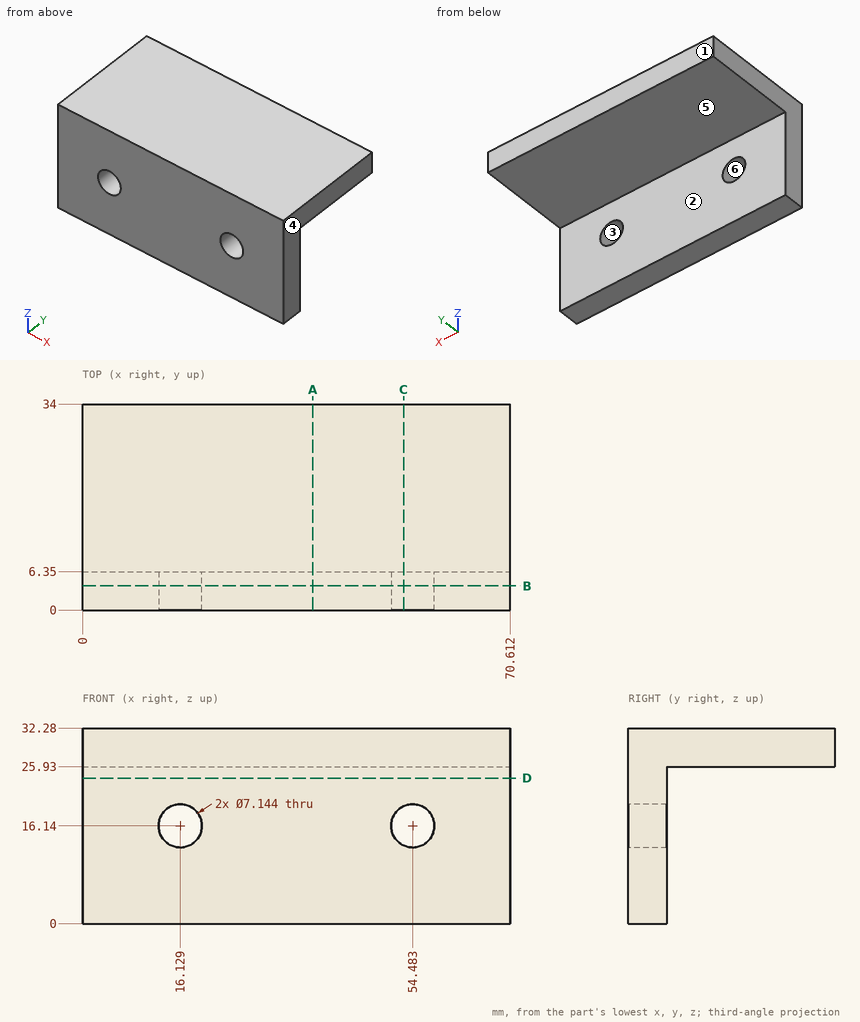
Geometry: see drawing. Coordinates: mm, zero at the bounding-box minimum. A direction names the side the tool comes from. Coordinates: 2 decimals unless noted, no trailing zeros. Loops run counter-clockwise (first coordinate to the right, second up) from the corner with the lowest first, then second, coordinate; pieces in that order, holes last. Notation, with made-up numbers: (-7, 89) - (52, 89) arc R9 cw to (52, 98) - close; hole circle Ø1 at (4, 35). An arc over 180 degrees is marked (long way). Answer in a Markdown table with one row per item.
(1) Cut plane D-D on z = 24. Output: boundary loops of the cut face in (x, y).
Model answer:
| item | result |
|---|---|
| outline | (0, 0) - (70.61, 0) - (70.61, 6.35) - (0, 6.35) - close |
(2) Mould query, pull axis X, two halves, no side actions, for the marked faces 3, 4, 5 and 6. Classes: pulls with the +X half, pulls with the -X half, needs draft (parallel to the pull), parting line crosses it, or undercut.
Model answer:
| item | result |
|---|---|
| face 3 | undercut |
| face 4 | pulls with the +X half |
| face 5 | needs draft |
| face 6 | undercut |
(3) Pin query (flat end, axial travel): P1, Ø9.5, axis at x = 54.48, z = 16.14, coming from the +Y side; P2, Ø8.5, axis at x = 28.5, y = 22, coming from the -Z side. Return the tip coordinate at first contact, or that it passes through.
Model answer:
| item | result |
|---|---|
| P1 | stops at y = 6.35 |
| P2 | stops at z = 25.93 |
(4) Cut plane B-B on y = 4. Output: boundary loops of the cut face in (x, z) (1 decimal).
Model answer:
| item | result |
|---|---|
| outline | (0, 0) - (70.6, 0) - (70.6, 32.3) - (0, 32.3) - close; hole circle Ø7.1 at (16.1, 16.1); hole circle Ø7.1 at (54.5, 16.1) |
(5) Set-up query: the marked faces 1 and 2. Return all of +Z, -Z, +X, -X, +Y, -Y with unobstructed straight access to the full face (end or side cutting, diameter ignored); none if empty.
Model answer:
| item | result |
|---|---|
| face 1 | +Z, -Z, +X, -X, +Y |
| face 2 | -Z, +X, -X, +Y |
(6) Cut plane A-A on x = 38. Output: boundary loops of the cut face in (y, z).
Model answer:
| item | result |
|---|---|
| outline | (0, 0) - (6.35, 0) - (6.35, 25.93) - (34, 25.93) - (34, 32.28) - (0, 32.28) - close |
(7) Material intervals for L1, parallel to Y at x = 44, z = 1; L2, parallel to Z at x = 4.5, y = 19.5, sorted ascending. Write a range as from..to.
Model answer:
| item | result |
|---|---|
| L1 | y = 0..6.35 |
| L2 | z = 25.93..32.28 |
(8) Cut plane C-C on x = 53. Output: boundary loops of the cut face in (y, z), plus the area to 3 significant figures.
Model answer:
| item | result |
|---|---|
| outline | (0, 0) - (6.35, 0) - (6.35, 12.89) - (0, 12.89) - close; (0, 19.39) - (6.35, 19.39) - (6.35, 25.93) - (34, 25.93) - (34, 32.28) - (0, 32.28) - close |
| area | 339 mm² |
